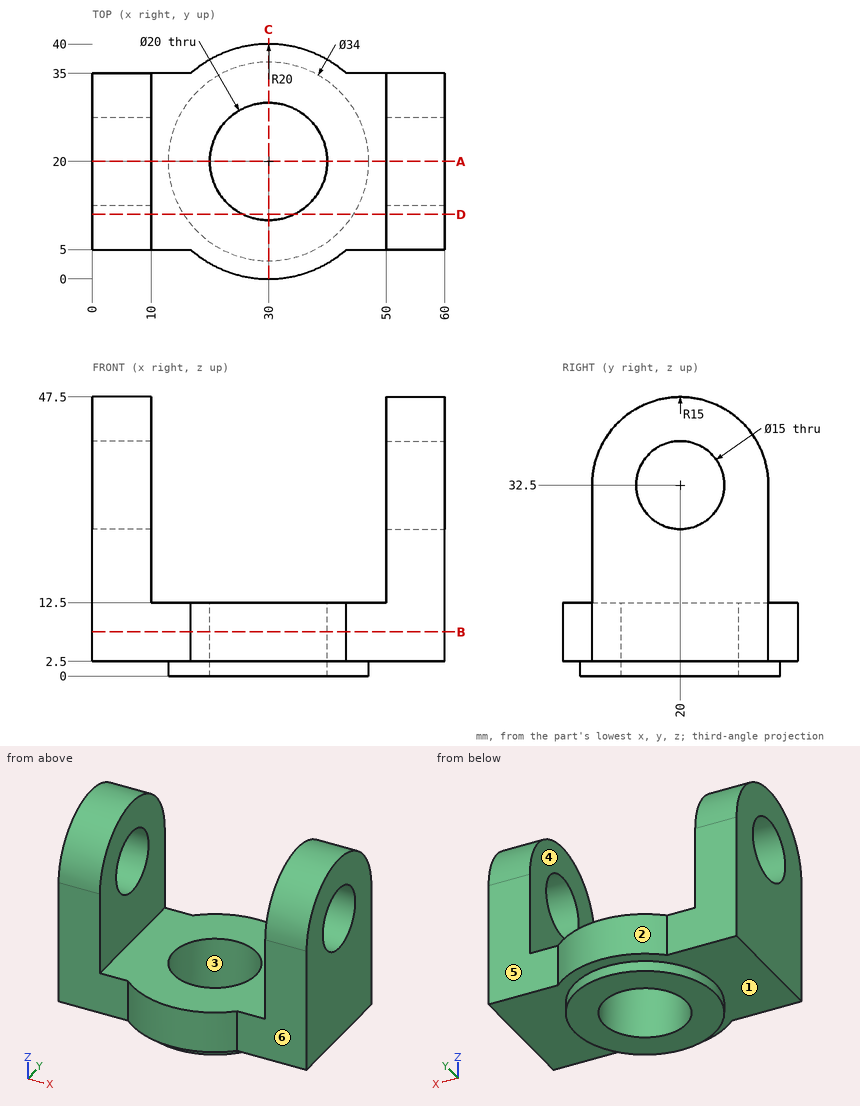
Job drawing, mm, ordinate dimensions from the low corner. One solid piece. A direction names the side the tool comes from. Round coordinates to 2 decimals unless told otherwise and drop trailing zeros. Write each loop counter-clockwise with the first axis right and the second up, starting at its lowest first coordinate (ties: lowest second). Pieces come first, ordered by that corner, then holes.
1) Mould opens along X. For the marked faces 1, 2 and 3 say: +X half, -X half, draft (parallel to the pull), parting line (faces both ways), or undercut.
2) Band-saw the part on D-D, the plane y = 11. List the corners of the cut face in (x, z), and give its area (3 significant figures).
3) Pin check, flat tips, straight feed: pin 1 (8.5 mm diameter, centred on x = 12.5, z = 17.5, fed in from -Y); pin 2 (8.5 mm diameter, centred on x = 10, z = 17, fed in from +Y); pin 3 (12 mm diameter, centred on x = 20.5, y = 23, fed in from +Z); pin 4 (4 mm diameter, centred on x = 31.5, z = 15, fed in from +Y). Stop position of each tip, or through.
4) 3-axis set-ups, long thin cutter, end or side, ignore diameter. For the marked faces 4, 5 and 6: which of +Z, -Z, +X, -X, +Y, -Y reach the whole face in a straight line?
5) Drill centre lines: probe 1 along Y at (x, z) = (52, 32); probe 2 along X at (y, z) = (32.5, 28); probe 3 along Z at (x, y) = (56.5, 20). Where is each one in solid material? Low to high.
6) Band-saw the part on B-B, the plane z = 7.5. List the corners of the cut face in (x, y), and give its area (3 significant figures).
7) Band-saw the part on A-A, the plane y = 20. List the corners of the cut face in (x, z).
8) Band-saw the part on C-C, the plane x = 30. List the corners of the cut face in (y, z).
Ans:
1. face 1: draft
1. face 2: parting line
1. face 3: undercut
2. outline: (0, 2.5) - (15.58, 2.5) - (15.58, 0) - (25.64, 0) - (25.64, 12.5) - (10, 12.5) - (10, 44.5) - (0, 44.5) - close; (34.36, 0) - (44.42, 0) - (44.42, 2.5) - (60, 2.5) - (60, 44.5) - (50, 44.5) - (50, 12.5) - (34.36, 12.5) - close
2. area: 1,200 mm2
3. pin 1: stops at y = 5
3. pin 2: stops at y = 35
3. pin 3: stops at z = 12.5
3. pin 4: passes through
4. face 4: +Z, +Y, -Y
4. face 5: +Z, -Z, +X, +Y
4. face 6: +Z, -Z, +X, -Y
5. probe 1: y = 5 to 12.52, 27.48 to 35
5. probe 2: x = 0 to 10, 50 to 60
5. probe 3: z = 2.5 to 25, 40 to 47.5
6. outline: (0, 5) - (16.77, 5) arc R20 ccw to (43.23, 5) - (60, 5) - (60, 35) - (43.23, 35) arc R20 ccw to (16.77, 35) - (0, 35) - close; hole circle Ø20 at (30, 20)
6. area: 1,670 mm2
7. outline: (0, 2.5) - (13, 2.5) - (13, 0) - (20, 0) - (20, 12.5) - (10, 12.5) - (10, 25) - (0, 25) - close; (0, 40) - (10, 40) - (10, 47.5) - (0, 47.5) - close; (40, 0) - (47, 0) - (47, 2.5) - (60, 2.5) - (60, 25) - (50, 25) - (50, 12.5) - (40, 12.5) - close; (50, 40) - (60, 40) - (60, 47.5) - (50, 47.5) - close
8. outline: (0, 2.5) - (3, 2.5) - (3, 0) - (10, 0) - (10, 12.5) - (0, 12.5) - close; (30, 0) - (37, 0) - (37, 2.5) - (40, 2.5) - (40, 12.5) - (30, 12.5) - close
